Geometry: final body of the model. Coordinates: model frame, mm. Coordinates: 2 decimals unless noted, no trailing zeros. Loops run counter-clockwise (first coordinate to the right, second up) from the corner with the lowest first, then second, coordinate; pieces in that order, holes last. Notation, with made-up numbers: (45.5, 16) - (53.5, 16) arc R9 ccw to (53.5, 33) - close; hole circle Ø1 at (66, -6). An arc over 180 degrees is marked (long way). Put each result on its own line as item: value. Start each with the question number.
1) Section A-A on z = -292.5. Output: boundary loops of the cut face in (x, y), and give its area (3 significant figures).
2) Contact query for flat-ended pins moving along their axis: pin 1 Ø10.5 at (x, z) = (14.986, -401.094) entering from +Y; pin 2 Ø6 at (x, z) = (14.986, -14.986) entering from -Y. Output: stop coordinate, or through.
3) Section C-C on y = 9.5. Output: boundary loops of the cut face in (x, z), and give its area (3 significant figures).
4) Section B-B on x = 254. Output: boundary loops of the cut face in (y, z).
5) Material intervals for line 1 along Z through (x, y) = (225, 7.75); line 2 along X through (y, z) = (0.5, -310), sorted ascending. Write a range as from..to.
```python
from build123d import *

# Parameters (mm, degrees)
SKETCH1_W                                  = 416.08
SKETCH1_H                                  = 416.08
BOSS_EXTRUDE1_DEPTH                        = 12.7
SKETCH2_R                                  = 3.683
CUT_EXTRUDE1_DEPTH                         = 589.563015148
SKETCH3_R                                  = 8.89
CUT_EXTRUDE2_DEPTH                         = 6.35
MIRROR1_AT_THE_SECOND_PLANE_COPY_1_SKETC_R = 3.683
MIRROR1_AT_THE_SECOND_PLANE_COPY_1_DEPTH   = 589.563015148
MIRROR1_AT_THE_SECOND_PLANE_COPY_2_SKETC_R = 8.89
MIRROR1_AT_THE_SECOND_PLANE_COPY_2_DEPTH   = 6.35
CUT_EXTRUDE3_REACH                         = 590.563
SKETCH4_W                                  = 112.243977319
SKETCH4_H                                  = 36.843442936


with BuildPart() as part:
    # Sketch1 → Boss-Extrude1 (new body)
    with BuildSketch(Plane(origin=(0, 0, 0), x_dir=(1, 0, 0), z_dir=(0, 1, 0))):
        with Locations((208.04, 208.04)):
            Rectangle(SKETCH1_W, SKETCH1_H)
    extrude(amount=BOSS_EXTRUDE1_DEPTH)

    # Sketch2 → Cut-Extrude1 (cut, through all)
    with BuildSketch(Plane(origin=(0, 12.7, 0), x_dir=(1, 0, 0), z_dir=(0, 1, 0))):
        with Locations(Location((14.986, 14.986, 0), (0, 0, 270))):
            Circle(SKETCH2_R)
    cut_extrude1 = extrude(amount=-CUT_EXTRUDE1_DEPTH, mode=Mode.SUBTRACT)

    # Sketch3 → Cut-Extrude2 (cut, symmetric)
    with BuildSketch(Plane(origin=(0, 12.7, 0), x_dir=(1, 0, 0), z_dir=(0, 1, 0))):
        with Locations(Location((14.986, 14.986, 0), (0, 0, 270))):
            Circle(SKETCH3_R)
    cut_extrude2 = extrude(amount=CUT_EXTRUDE2_DEPTH, both=True, mode=Mode.SUBTRACT)

    # Mirror1: Cut-Extrude1, Cut-Extrude2 across plane
    add(cut_extrude1.mirror(Plane(origin=(0, 0, -208.04), x_dir=(1, 0, 0), z_dir=(0, 0, -1))), mode=Mode.SUBTRACT)
    add(cut_extrude2.mirror(Plane(origin=(0, 0, -208.04), x_dir=(1, 0, 0), z_dir=(0, 0, -1))), mode=Mode.SUBTRACT)

    # Mirror1 at the second plane: Cut-Extrude1, Cut-Extrude2 across plane
    add(cut_extrude1.mirror(Plane.ZY.offset(-208.04)), mode=Mode.SUBTRACT)
    add(cut_extrude2.mirror(Plane.ZY.offset(-208.04)), mode=Mode.SUBTRACT)

    # Mirror1 at the second plane copy 1 sketc → Mirror1 at the second plane copy 1 (cut, through all)
    with BuildSketch(Plane(origin=(416.08, 12.7, -416.08), x_dir=(-1, 0, 0), z_dir=(0, 1, 0))):
        with Locations(Location((14.986, 14.986, 0), (0, 0, 270))):
            Circle(MIRROR1_AT_THE_SECOND_PLANE_COPY_1_SKETC_R)
    extrude(amount=-MIRROR1_AT_THE_SECOND_PLANE_COPY_1_DEPTH, mode=Mode.SUBTRACT)

    # Mirror1 at the second plane copy 2 sketc → Mirror1 at the second plane copy 2 (cut, symmetric)
    with BuildSketch(Plane(origin=(416.08, 12.7, -416.08), x_dir=(-1, 0, 0), z_dir=(0, 1, 0))):
        with Locations(Location((14.986, 14.986, 0), (0, 0, 270))):
            Circle(MIRROR1_AT_THE_SECOND_PLANE_COPY_2_SKETC_R)
    extrude(amount=MIRROR1_AT_THE_SECOND_PLANE_COPY_2_DEPTH, both=True, mode=Mode.SUBTRACT)

    # Sketch4 → Cut-Extrude3 (cut, up to next)
    with BuildSketch(Plane.XZ, mode=Mode.PRIVATE) as cut_extrude3_sk1:
        with Locations((207.758599761, -296.609069082)):
            Rectangle(SKETCH4_W, SKETCH4_H)
    cut_extrude3_tool1 = extrude(cut_extrude3_sk1.sketch, amount=-CUT_EXTRUDE3_REACH, mode=Mode.PRIVATE) & part.part
    add(cut_extrude3_tool1.solids().sort_by_distance((207.7586, 0, -296.609069))[0], mode=Mode.SUBTRACT)


solid = part.part
```
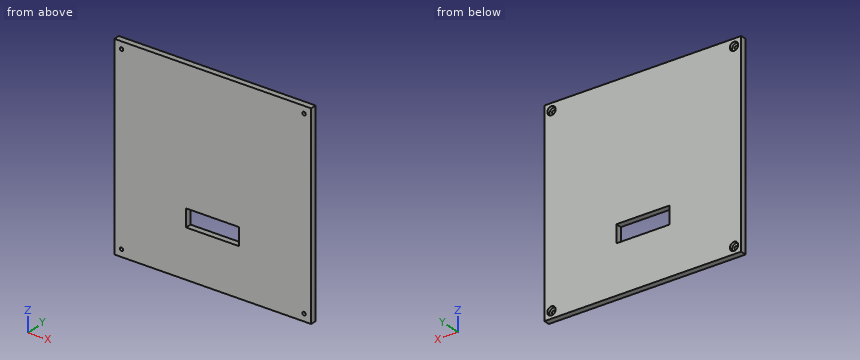
Answer block:
1. outline: (0, 0) - (151.64, 0) - (151.64, 12.7) - (0, 12.7) - close; (263.88, 0) - (416.08, 0) - (416.08, 12.7) - (263.88, 12.7) - close
1. area: 3,860 mm²
2. pin 1: stops at y = 6.35
2. pin 2: passes through
3. outline: (0, -416.08) - (416.08, -416.08) - (416.08, 0) - (0, 0) - close; hole circle Ø17.78 at (14.99, -401.09); hole circle Ø17.78 at (14.99, -14.99); hole (151.64, -315.03) - (263.88, -315.03) - (263.88, -278.19) - (151.64, -278.19) - close; hole circle Ø17.78 at (401.09, -401.09); hole circle Ø17.78 at (401.09, -14.99)
3. area: 168,000 mm²
4. outline: (0, -416.08) - (12.7, -416.08) - (12.7, -315.03) - (0, -315.03) - close; (0, -278.19) - (12.7, -278.19) - (12.7, 0) - (0, 0) - close
5. line 1: z = -416.08..-315.03, -278.19..0
5. line 2: x = 0..151.64, 263.88..416.08
